from build123d import *

# Parameters (mm, degrees)
SKETCH1_R          = 85
BASE_FLANGE1_DEPTH = 3
SKETCH2_R          = 4.6
EXTRUDE1_DEPTH     = 3
SKETCH3_R          = 4.6
EXTRUDE2_DEPTH     = 3
CIRPATTERN1_COUNT  = 8
SKETCH4_R          = 2.1
CUT_EXTRUDE1_DEPTH = 10


# Sheet-metal steps are written as plain solids
with BuildPart() as part:
    # Sketch1 → Base-Flange1 (new body)
    with BuildSketch(Plane.XY):
        with BuildLine():
            Line((168, 168), (168, 225))
            Line((168, 225), (128, 225))
            Line((128, 225), (128, 195))
            ThreePointArc((128, 195), (0, 155.04323819), (-128, 195))
            Line((-128, 195), (-128, 225))
            Line((-128, 225), (-168, 225))
            Line((-168, 225), (-168, 168))
            Line((-168, 168), (-225, 168))
            Line((-225, 168), (-225, 128))
            Line((-225, 128), (-195, 128))
            ThreePointArc((-195, 128), (-155.04323819, 0), (-195, -128))
            Line((-195, -128), (-225, -128))
            Line((-225, -128), (-225, -168))
            Line((-225, -168), (-168, -168))
            Line((-168, -168), (-168, -225))
            Line((-168, -225), (-128, -225))
            Line((-128, -225), (-128, -195))
            ThreePointArc((-128, -195), (0, -155.04323819), (128, -195))
            Line((128, -195), (128, -225))
            Line((128, -225), (168, -225))
            Line((168, -225), (168, -168))
            Line((168, -168), (225, -168))
            Line((225, -168), (225, -128))
            Line((225, -128), (195, -128))
            ThreePointArc((195, -128), (155.04323819, 0), (195, 128))
            Line((195, 128), (225, 128))
            Line((225, 128), (225, 168))
            Line((225, 168), (168, 168))
        make_face()
        Circle(SKETCH1_R, mode=Mode.SUBTRACT)
    extrude(amount=BASE_FLANGE1_DEPTH)

    # Sketch2 → Extrude1 (cut)
    with BuildSketch(Plane.XY.offset(3)):
        with Locations((148, 212.5)):
            Circle(SKETCH2_R)
        with Locations((148, 182.5)):
            Circle(SKETCH2_R)
        with Locations((182.5, 148)):
            Circle(SKETCH2_R)
        with Locations((212.5, 148)):
            Circle(SKETCH2_R)
        with Locations(Location((212.5, -148, 0), (0, 0, 180))):
            Circle(SKETCH2_R)
        with Locations(Location((182.5, -148, 0), (0, 0, 180))):
            Circle(SKETCH2_R)
        with Locations(Location((148, -182.5, 0), (0, 0, 180))):
            Circle(SKETCH2_R)
        with Locations(Location((148, -212.5, 0), (0, 0, 180))):
            Circle(SKETCH2_R)
        with Locations((-148, -212.5)):
            Circle(SKETCH2_R)
        with Locations((-148, -182.5)):
            Circle(SKETCH2_R)
        with Locations((-182.5, -148)):
            Circle(SKETCH2_R)
        with Locations((-212.5, -148)):
            Circle(SKETCH2_R)
        with Locations(Location((-212.5, 148, 0), (0, 0, 180))):
            Circle(SKETCH2_R)
        with Locations(Location((-182.5, 148, 0), (0, 0, 180))):
            Circle(SKETCH2_R)
        with Locations(Location((-148, 182.5, 0), (0, 0, 180))):
            Circle(SKETCH2_R)
        with Locations(Location((-148, 212.5, 0), (0, 0, 180))):
            Circle(SKETCH2_R)
    extrude(amount=-EXTRUDE1_DEPTH, mode=Mode.SUBTRACT)

    # Sketch3 → Extrude2 (cut)
    with BuildSketch(Plane.XY.offset(3)):
        with Locations((0, 95)):
            Circle(SKETCH3_R)
    extrude2 = extrude(amount=-EXTRUDE2_DEPTH, mode=Mode.SUBTRACT)

    # CirPattern1: Extrude2 ×8 about axis
    cirpattern1_axis = Axis((0, 0, 0), (0, 0, 1))
    for i in range(1, CIRPATTERN1_COUNT):
        add(extrude2.rotate(cirpattern1_axis, i * 360 / CIRPATTERN1_COUNT), mode=Mode.SUBTRACT)

    # Sketch4 → Cut-Extrude1 (cut)
    with BuildSketch(Plane.XY.offset(3)):
        with Locations((-146.786796564, -146.786796564)):
            Circle(SKETCH4_R)
        with Locations((-128.402020254, -128.402020254)):
            Circle(SKETCH4_R)
        with Locations((-90.925360851, -90.925360851)):
            Circle(SKETCH4_R)
        with Locations((130.523340597, -130.523340597)):
            Circle(SKETCH4_R)
        with Locations((146.786796564, -146.786796564)):
            Circle(SKETCH4_R)
    extrude(amount=-CUT_EXTRUDE1_DEPTH, mode=Mode.SUBTRACT)


solid = part.part
Read the model definition and answer for the solid it produces. Units are mm, in the model's axes. Give positions to 0.01 mm unless a question says otherwise; leave off trailing zeros. Loops run counter-clockwise (first coordinate to the right, second up) from the corner with the lowest first, then second, coordinate; pieces in that order, holes last. Notation, with made-up numbers: M 42.5,2.25 L 58.5,2.25 A17 cw 58.5,27.25 Z; hole C 81,0.25 d1. An arc over 180 degrees is marked long. Write each question's results on one line, items separated by ' | '.
1. Section C-C on z = 2.5 is taken. State how many separate pieces and enclosed holes the cut face has, plus the area to 3 significant figures.
Values:
separate pieces: 1 | enclosed holes: 30 | area: 107,000 mm^2
2. The mould has two halves that part along X. Classify faces 1 (the face through (-1.91, -155.05, 1.48)), 2 (the face through (155.05, -1.91, 1.48)), 3 (the face through (-103, 3, 0)): pulls with the +X half, pulls with the -X half, needs draft (parallel to the pull), parting line crosses it, or undercut.
Values:
face 1: undercut | face 2: pulls with the +X half | face 3: needs draft
3. Section B-B on y = 77 is taken. Give the vertices of the cut face in (x, z), plus the area to 3 significant figures.
Values:
outline: M -168.63,0 L -36,0 L -36,3 L -168.63,3 Z; M 36,0 L 168.63,0 L 168.63,3 L 36,3 Z | area: 796 mm^2
4. Straight lines are drawn through the part: line 1 (Y direction, x = 0, z = 1.75); line 2 (Y direction, x = 199.5, z = 0.6); line 3 (X direction, y = 189, z = 2.05). For each, find the intervals that lie inside material, in ascending order. Write a range as [from, to].
Values:
line 1: y = [-155.04, -99.6], [-90.4, -85], [85, 90.4], [99.6, 155.04] | line 2: y = [-168, -128], [128, 168] | line 3: x = [-168, -118.86], [118.86, 168]
5. Section D-D on x = -116.5 is taken. Give the vertices of the cut face in (y, z), plus the area to 3 significant figures.
Values:
outline: M -187.55,0 L 187.55,0 L 187.55,3 L -187.55,3 Z | area: 1,130 mm^2
6. Section A-A on x = -34.5 is taken. Give the vertices of the cut face in (y, z).
Values:
outline: M -157.7,0 L -77.68,0 L -77.68,3 L -157.7,3 Z; M 77.68,0 L 157.7,0 L 157.7,3 L 77.68,3 Z
7. Given pin 1 (1 mm diameter, centred on x = 83.5, z = 2.5, fed in from -Y); pin 2 (1.5 mm diameter, centred on x = 196.5, z = 1, fed in from -Y), each flat-ended and moving along its own axis, determine where each tip first touches the part or whether it passes through.
Values:
pin 1: stops at y = -171.31 | pin 2: stops at y = -168
